from build123d import *

# Parameters (mm, degrees)
EXTRUDE_1_DEPTH = 6
SKETCH_2_R      = 4
EXTRUDE_2_DEPTH = 40
FILLET_3_R      = 0.2


with BuildPart() as part:
    # 草图1 → 凸台-拉伸1 (new body)
    with BuildSketch(Plane.XY):
        Polygon((0, 7.967433715), (-6.9, 3.983716857), (-6.9, -3.983716857), (0, -7.967433715), (6.9, -3.983716857), (6.9, 3.983716857), align=None)
    extrude(amount=-EXTRUDE_1_DEPTH)

    # 草图2 → 凸台-拉伸2 (add)
    with BuildSketch(Plane(origin=(0, 0, -6), x_dir=(-1, 0, 0), z_dir=(0, 0, -1))):
        Circle(SKETCH_2_R)
    extrude(amount=EXTRUDE_2_DEPTH)

    # 草图3 → 切除-旋转1 (revolve, cut)
    with BuildSketch(Plane(origin=(0, 0, 0), x_dir=(0, 0, -1), z_dir=(1, 0, 0))):
        Polygon((0, -6.917433715), (1.05, -7.967433715), (0, -7.967433715), align=None)
        Polygon((6, -6.917433715), (4.95, -7.967433715), (6, -7.967433715), align=None)
    revolve(axis=Axis((0, 0, 0), (0, 0, 1)), mode=Mode.SUBTRACT)

    # 圆角3
    fillet_3_edges = [part.edges().sort_by_distance(p)[0] for p in [
        (4, 0, -46),
    ]]
    fillet(fillet_3_edges, radius=FILLET_3_R)


solid = part.part
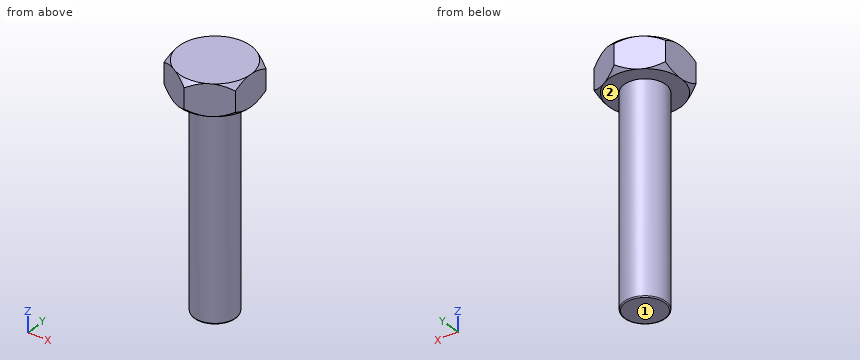
Geometry: final body of the model. Coordinates: model frame, mm. Face numbers are marked on the shaded views. A direction names the side the tool comes from. Round coordinates to 2 decimals unless told otherwise and drop trailing zeros. Order: outer loops, then holes, each group sorted by start corner. A loop starts at its lowest first (then second) coordinate and runs counter-clockwise, first axis right, second up. Notation, with made-up numbers: (64.25, 42.5) -> (84.25, 42.5) arc R36 ccw to (84.25, 80.5) -> close; hole circle Ø1 at (58.25, -36). An arc over 180 degrees is marked (long way). Put each result on its own line as item: value. Start each with the question number.
Q1. Line query: probe 1 along Z at (x, y) = (4.25, -4.5); probe 2 along X at (y, z) = (1.25, -21). Output: solid intervals per line, ascending.
Q2. Section A-A on y = 0. Return the cut outline in (x, z), and give its area (3 significant figures).
Q3. Section B-B on z = -21. Return the cut outline in (x, y).
Q4. First-contact query: pin 1 (1.5 mm diameter, centred on x = 1.5, z = -23, fed in from +Y); pin 2 (3 mm diameter, centred on x = 0.5, y = 6, fed in from -Z); pin 3 (8 mm diameter, centred on x = -2.5, z = -38, fed in from +Y). Flat tips, straight axial feed; report the tip coordinate or a pass-through.
Q5. Reachability of the marked faces 1 and 2 from +Z, -Z, +X, -X, +Y, -Y: full face, straight path, thin tool, end or side. Return the list, or none.
Ans:
1. probe 1: z = -6 to 0
1. probe 2: x = -3.8 to 3.8
2. outline: (-6.9, -6) -> (-4, -6) -> (-4, -45.8) arc R0.2 ccw to (-3.8, -46) -> (3.8, -46) arc R0.2 ccw to (4, -45.8) -> (4, -6) -> (6.9, -6) -> (6.9, 0) -> (-6.9, 0) -> close
2. area: 403 mm2
3. outline: circle Ø8 at (0, 0)
4. pin 1: stops at y = 3.93
4. pin 2: stops at z = -6
4. pin 3: stops at y = 4
5. face 1: -Z, +X, -X, +Y, -Y
5. face 2: -Z
